```python
from build123d import *

# Parameters (mm, degrees)
SKETCH1_W           = 300
SKETCH1_H           = 30
BOSS_EXTRUDE1_DEPTH = 14
SKETCH2_R           = 3
CUT_EXTRUDE1_DEPTH  = 14
FILLET1_R           = 10


with BuildPart() as part:
    # Sketch1 → Boss-Extrude1 (new body)
    with BuildSketch(Plane.XY):
        Rectangle(SKETCH1_W, SKETCH1_H)
    extrude(amount=BOSS_EXTRUDE1_DEPTH)

    # Sketch2 → Cut-Extrude1 (cut)
    with BuildSketch(Plane.XY.offset(14)):
        with Locations((100, 0)):
            Circle(SKETCH2_R)
        with Locations((-100, 0)):
            Circle(SKETCH2_R)
        with Locations((-140, 0)):
            Circle(SKETCH2_R)
        with Locations((-120, 0)):
            Circle(SKETCH2_R)
        with Locations((120, 0)):
            Circle(SKETCH2_R)
        with Locations((140, 0)):
            Circle(SKETCH2_R)
        with Locations((-80, 0)):
            Circle(SKETCH2_R)
        with Locations((80, 0)):
            Circle(SKETCH2_R)
        with Locations((-60, 0)):
            Circle(SKETCH2_R)
        with Locations((-40, 0)):
            Circle(SKETCH2_R)
        with Locations((60, 0)):
            Circle(SKETCH2_R)
        with Locations((40, 0)):
            Circle(SKETCH2_R)
        with Locations((-20, 0)):
            Circle(SKETCH2_R)
        Circle(SKETCH2_R)
        with Locations((20, 0)):
            Circle(SKETCH2_R)
    extrude(amount=-CUT_EXTRUDE1_DEPTH, mode=Mode.SUBTRACT)

    # Fillet1
    fillet1_edges = [part.edges().sort_by_distance(p)[0] for p in [
        (150, -15, 7),
        (-150, -15, 7),
        (-150, 15, 7),
        (150, 15, 7),
    ]]
    fillet(fillet1_edges, radius=FILLET1_R)


solid = part.part
```
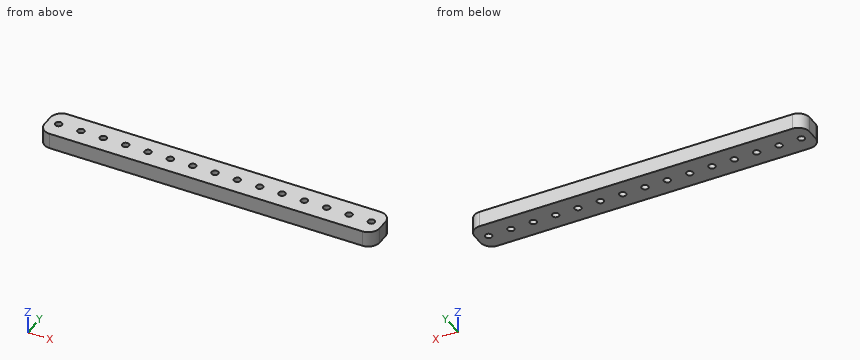
Check sheet for the modelled part. Datum: model origin and axes. Units: mm. Round coordinates to 2 decimals unless told otherwise and drop trailing zeros. Order: outer loops, then holes, each group sorted by start corner. A loop starts at its lowest first (then second) coordinate and runs counter-clockwise, first axis right, second up.
1) Section check B-B (z = 5.75). Give the number of separate pieces and of enclosed holes in the cut face, and give its area (3 significant figures).
2) Go/stop test with flat-tipped pins: pin 1 Ø5 at (x, y) = (-140, 0) entering from +Z; pin 2 Ø1.5 at (y, z) = (7, 7) entering from +X. Record where each tip stops, or that it passes through.
3) Scan lines: line 1 (Y direction, x = -100, z = 10.75); line 2 (Y direction, x = -82, z = 8.25); line 3 (X direction, y = 12.5, z = 11.5). Record each from-to range of solid material in increasing order.
4) Section check A-A (x = -40). Record the boundary of the cut face in (y, z), and give its area (3 significant figures).
Result:
1. separate pieces: 1
1. enclosed holes: 15
1. area: 8,490 mm2
2. pin 1: passes through
2. pin 2: stops at x = 149.92
3. line 1: y = -15 to -3, 3 to 15
3. line 2: y = -15 to -2.24, 2.24 to 15
3. line 3: x = -146.61 to 146.61
4. outline: (-15, 0) - (-3, 0) - (-3, 14) - (-15, 14) - close; (3, 0) - (15, 0) - (15, 14) - (3, 14) - close
4. area: 336 mm2
